Answer from the drawing. Dimensions are ordinates in mm from the lowest x, y and z of the part. A direction names the side the tool comes from. Give positions to 0.01 mm unless a question says otherwise; leave off trailing zeros. Write each loop counter-clockwise with the first axis right and the second up, starting at its lowest first coordinate (ties: lowest second). Pieces come first, ordered by that corner, then holes. Notation, with made-up numbers: (-39, 81.25) -> (-3, 81.25) arc R35 ccw to (-3, 120.25) -> close; hole circle Ø4 at (4, -13). An arc over 180 degrees is marked (long way). Put each result on its own line as item: value. Start each with the question number.
1) A cutting plane is placed at A-A (x = 31.1). Write down the section's boundary in (y, z) (3 decimals).
2) For the marked faces 1, 2 and 3, determine the directions among +Z, -Z, +X, -X, +Y, -Y from which every point of the face is accessible in a straight line to the end or side of a thin tool.
3) A cutting plane is placed at B-B (z = 34). Write down the section's boundary in (x, y) (3 decimals).
4) Flat-ended cylindrical pins translate along their axes: pin 1 Ø9 at (y, z) = (22.5, 20) entering from +X; pin 2 Ø10 at (x, z) = (29.5, 14.5) entering from -Y; pin 3 Ø12.5 at (x, y) = (33.5, 13.5) entering from -Z. Find the tip coordinate at first contact, or state that the pin passes through.
5) Find the intervals of material crossed by line 1 along Y through (x, z) = (31, 36); line 2 along Y through (x, z) = (159, 16.5); line 3 along X through (y, z) = (11.5, 8), in increasing order. Write a range as from..to.
6) A cutting plane is placed at C-C (y = 21.1). Write down the section's boundary in (x, z) (3 decimals).
7) For a pull along X with two mould halves and no side action, classify the marked faces 4, 5 and 6 as released by +X, released by -X, zero draft, split by the parting line, or undercut.
8) A cutting plane is placed at D-D (z = 22). Write down the section's boundary in (x, y), then the cut area to 3 significant figures.
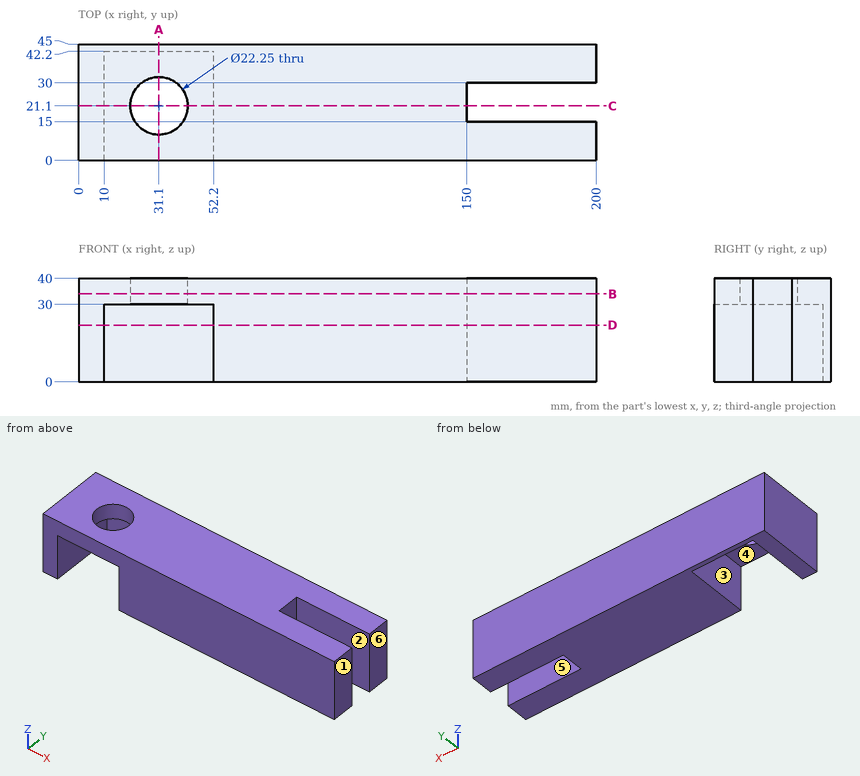
Reply:
1. outline: (0, 30) -> (9.975, 30) -> (9.975, 40) -> (0, 40) -> close; (32.225, 30) -> (42.2, 30) -> (42.2, 0) -> (45, 0) -> (45, 40) -> (32.225, 40) -> close
2. face 1: +Z, -Z, +X, +Y, -Y
2. face 2: +Z, -Z, +X
2. face 3: -Z, -Y
3. outline: (0, 0) -> (200, 0) -> (200, 15) -> (150, 15) -> (150, 30) -> (200, 30) -> (200, 45) -> (0, 45) -> close; hole circle Ø22.25 at (31.1, 21.1)
4. pin 1: stops at x = 150
4. pin 2: stops at y = 42.2
4. pin 3: stops at z = 30
5. line 1: y = 0..9.98, 32.22..45
5. line 2: y = 0..15, 30..45
5. line 3: x = 0..10, 52.2..200
6. outline: (0, 0) -> (10, 0) -> (10, 30) -> (19.975, 30) -> (19.975, 40) -> (0, 40) -> close; (42.225, 30) -> (52.2, 30) -> (52.2, 0) -> (150, 0) -> (150, 40) -> (42.225, 40) -> close
7. face 4: undercut
7. face 5: zero draft
7. face 6: released by +X
8. outline: (0, 0) -> (10, 0) -> (10, 42.2) -> (52.2, 42.2) -> (52.2, 0) -> (200, 0) -> (200, 15) -> (150, 15) -> (150, 30) -> (200, 30) -> (200, 45) -> (0, 45) -> close
8. area: 6,470 mm2
